The figure shows three views and two pictorial views of one solid part (mm, origin at its lowest corner). Answer the questions. Round coordinates to 2 decimals unless told otherwise and drop trailing zeros. Order: outer loops, then holes, each group sorted by start corner. A loop starts at its lowest first (then second) coordinate and runs counter-clockwise, first axis right, second up. Notation, with made-up numbers: (76.25, 76.25) - (92.25, 76.25) arc R21 ccw to (92.25, 90.25) - close; hole circle Ø6 at (86.25, 70.5). An arc over 180 degrees is marked (long way). Use CSV: the item, a comma, the result in double quotes. Start each with the question number.
Item 1: Straight lines are drawn through the part: line 1 along Y through (x, z) = (16, 3.1); line 2 along X through (y, z) = (2.75, 3.55); line 3 along X through (y, z) = (3.25, 1.3). For each, find the intervals that lie inside material, in ascending order. Write a range as [from, to].
Item 2: Determine the mould class of the marked faces 1, 2 and 3 for opening direction X: +X half, -X half, draft (parallel to the pull), parting line (faces both ways), or undercut.
Item 3: Find section A-A, the plane z = 0.3. Give the vertices of the cut face in (x, y), plus the area to 3 significant figures.
Item 4: Find section C-C, the plane y = 16. Give the vertices of the cut face in (x, z), plus the area to 3 significant figures.
Item 5: Find section D-D, the plane z = 3.9. Give the vertices of the cut face in (x, y), plus the area to 3 significant figures.
Item 6: Find section B-B, the plane x = 4. Give the vertices of the cut face in (y, z), plus the area to 3 significant figures.
Item 7: A flat-ended cylindrical pin translates along its axis: P1, Ø3.5, axis at x = 4, y = 16, coming from the +Z side. Find the tip coordinate at first contact, or state that the pin passes through.
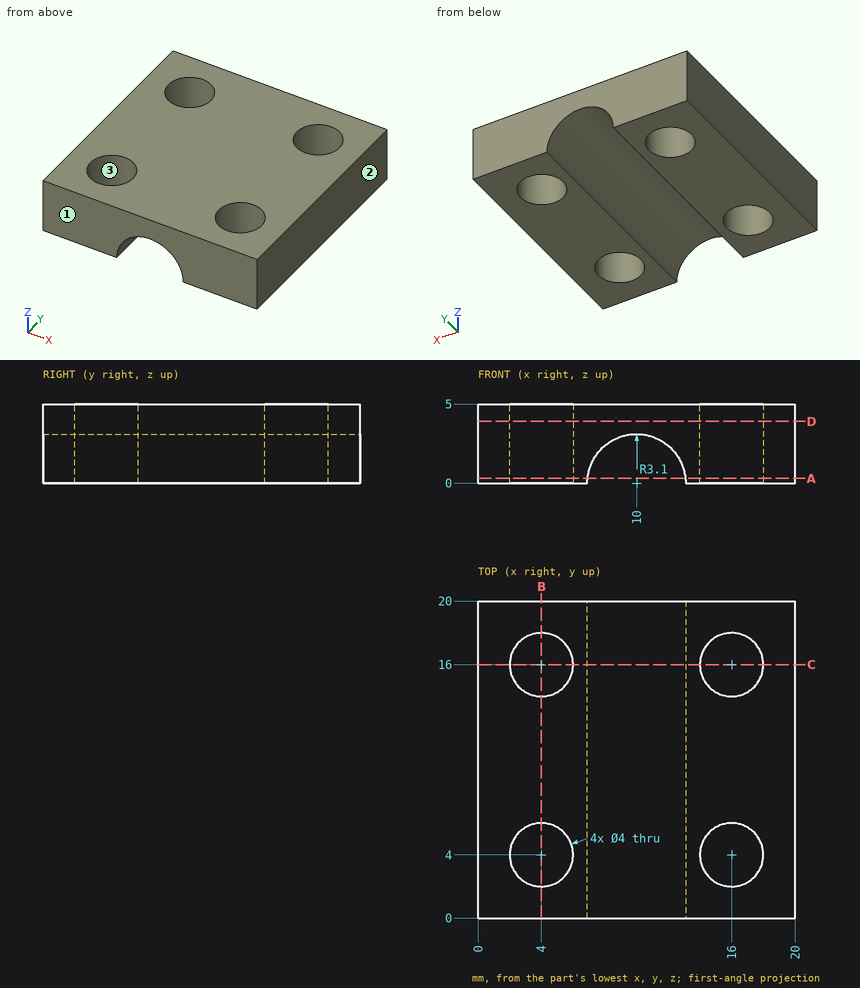
Worked out:
1,line 1,"y = [0, 2], [6, 14], [18, 20]"
1,line 2,"x = [0, 2.44], [5.56, 14.44], [17.56, 20]"
1,line 3,"x = [0, 2.15], [5.85, 7.19], [12.81, 14.15], [17.85, 20]"
2,face 1,"draft"
2,face 2,"+X half"
2,face 3,"undercut"
3,outline,"(0, 0) - (6.91, 0) - (6.91, 20) - (0, 20) - close; (13.09, 0) - (20, 0) - (20, 20) - (13.09, 20) - close; hole circle Ø4 at (4, 4); hole circle Ø4 at (4, 16); hole circle Ø4 at (16, 4); hole circle Ø4 at (16, 16)"
3,area,"226 mm²"
4,outline,"(0, 0) - (2, 0) - (2, 5) - (0, 5) - close; (6, 0) - (6.9, 0) arc R3.1 cw to (13.1, 0) - (14, 0) - (14, 5) - (6, 5) - close; (18, 0) - (20, 0) - (20, 5) - (18, 5) - close"
4,area,"44.9 mm²"
5,outline,"(0, 0) - (20, 0) - (20, 20) - (0, 20) - close; hole circle Ø4 at (4, 4); hole circle Ø4 at (4, 16); hole circle Ø4 at (16, 4); hole circle Ø4 at (16, 16)"
5,area,"350 mm²"
6,outline,"(0, 0) - (2, 0) - (2, 5) - (0, 5) - close; (6, 0) - (14, 0) - (14, 5) - (6, 5) - close; (18, 0) - (20, 0) - (20, 5) - (18, 5) - close"
6,area,"60.0 mm²"
7,P1,"passes through"
